Read the model definition and answer for the solid it produces. Units are mm, in the model's axes. Give positions to 0.01 mm unless a question says otherwise; leave off trailing zeros. Order: outer loops, then holes, each group sorted by start corner. A loop starts at its lowest first (then second) coordinate and runs counter-clockwise, first axis right, second up.
Item 1: A cutting plane is placed at A-A (x = 0). Write down the section's boundary in (y, z) (3 decimals).
Item 2: A cutting plane is placed at C-C (y = 8). Write down the section's boundary in (x, z).
Item 3: A cutting plane is placed at B-B (y = 4.25). Write down the section's boundary in (x, z).
Item 4: Given pin 1 Ø1 at (y, z) = (8.5, 3) entering from -X; pin 2 Ø2 at (y, z) = (11, -2.5) entering from -X; pin 3 Ø5 at (y, z) = (6.5, -3.5) entering from +X, each flat-ended and moving along its own axis, determine where each tip first touches the part or whether it passes through.
Item 5: Find the intervals of material crossed by line 1 along X through (y, z) = (10.75, 4.5); line 2 along Z through (x, y) = (2.75, 2); line 3 along Z through (x, y) = (-3.5, 9.25), in increasing order.
from build123d import *

# Parameters (mm, degrees)
SKETCH1_R           = 8
BOSS_EXTRUDE1_DEPTH = 2
SKETCH2_R           = 6
BOSS_EXTRUDE2_DEPTH = 12
BOSS_EXTRUDE2_TAPER = 3
FILLET1_R           = 1.016
CHAMFER1_SIZE       = 1.905
CHAMFER1_SIZE2      = 2.013117328
FILLET3_R           = 1.016


with BuildPart() as part:
    # Sketch1 → Boss-Extrude1 (new body)
    with BuildSketch(Plane(origin=(0, 0, 0), x_dir=(1, 0, 0), z_dir=(0, 1, 0))):
        with Locations(Location((0, 0, 0), (0, 0, 270))):
            Circle(SKETCH1_R)
    extrude(amount=BOSS_EXTRUDE1_DEPTH)

    # Sketch2 → Boss-Extrude2 (add)
    with BuildSketch(Plane(origin=(0, 2, 0), x_dir=(1, 0, 0), z_dir=(0, 1, 0))):
        Circle(SKETCH2_R)
    extrude(amount=BOSS_EXTRUDE2_DEPTH, taper=BOSS_EXTRUDE2_TAPER)

    # Fillet1
    fillet1_edges = [part.edges().sort_by_distance(p)[0] for p in [
        (-5.371106649, 14, 0),
    ]]
    fillet(fillet1_edges, radius=FILLET1_R)

    # Chamfer1
    chamfer1_edges = [part.edges().sort_by_distance(p)[0] for p in [
        (-6, 2, 0),
    ]]
    chamfer1_side = [part.faces().sort_by_distance(p)[0] for p in [
        (0, 2, -7.77372583),
    ]]
    chamfer(chamfer1_edges, length=CHAMFER1_SIZE, length2=CHAMFER1_SIZE2, reference=chamfer1_side[0])

    # Fillet3
    # the kernel refuses this fillet: 1.016 mm, written as the material it takes off along each edge
    with BuildSketch(Plane(origin=(0, 2, 0), x_dir=(0, 0, 1), z_dir=(-1, 0, 0))) as fillet3_piece_1:
        with BuildLine():
            CenterArc((6.984, -0.428969696), FILLET3_R, 0, 24.97446259)
            Line((8, -0.428969696), (8.02032, -0.428969696))
            Line((8.02032, -0.428969696), (8.02032, 0))
            Line((8.02032, 0), (8, 0.02032))
            ThreePointArc((8, 0.02032), (7.9525, 0.02032), (7.92342, 0.008579394))
            Line((7.92342, 0.008579394), (7.905, 0))
        make_face()
    revolve(axis=Axis((0, 2, 0), (0, 1, 0)), mode=Mode.SUBTRACT)


solid = part.part
Response values:
1. outline: (0, -8) - (1.571, -8) arc R1.016 ccw to (2, -7.905) - (4.01, -5.895) - (13.037, -5.422) arc R1.016 ccw to (14, -4.407) - (14, 4.407) arc R1.016 ccw to (13.037, 5.422) - (4.01, 5.895) - (2, 7.905) arc R1.016 ccw to (1.571, 8) - (0, 8) - close
2. outline: circle Ø11.37 at (0, 0)
3. outline: circle Ø11.76 at (0, 0)
4. pin 1: stops at x = -5.08
4. pin 2: stops at x = -5.33
4. pin 3: stops at x = 5.7
5. line 1: x = -3.23 to 3.23
5. line 2: z = -7.41 to 7.41
5. line 3: z = -4.4 to 4.4
